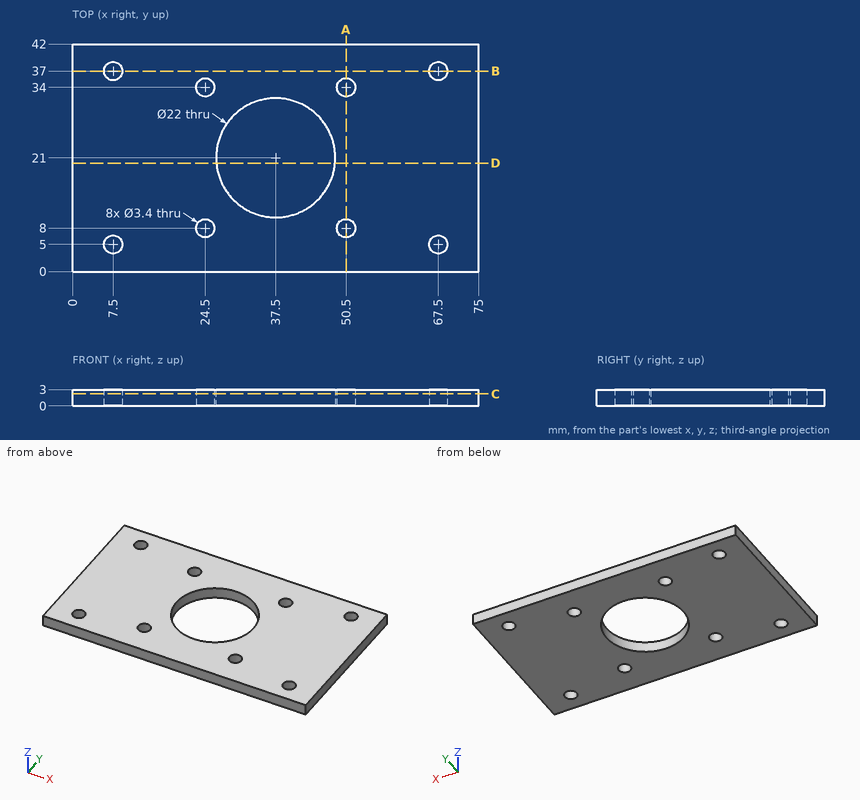
Check sheet for the drawn part. Datum: minimum x, y, z corner. Units: mm. Coordinates: 2 decimals unless noted, no trailing zeros. Loops run counter-clockwise (first coordinate to the right, second up) from the corner with the lowest first, then second, coordinate; pieces in that order, holes last. Notation, with made-up numbers: (40.25, 63.25) -> (51.25, 63.25) arc R27 cw to (51.25, 84.25) -> close; hole circle Ø2 at (4.25, -36). An arc over 180 degrees is marked (long way). Write each question's results on one line, items separated by ' | '.
Item 1: Section check C-C, the plane z = 2.2. Count the separate pieces of the cut face and the enclosed holes in it, plus the area to 3 significant figures.
Found:
separate pieces: 1 | enclosed holes: 9 | area: 2,700 mm2
Item 2: Material ranges on L1, parallel to Y at x = 67.5, z = 1.55; L2, parallel to Y at x = 50.5, z = 0.8; L3, parallel to X at y = 6.5, z = 2.85, recorded low to high.
Found:
L1: y = 0 to 3.3, 6.7 to 35.3, 38.7 to 42 | L2: y = 0 to 6.3, 9.7 to 32.3, 35.7 to 42 | L3: x = 0 to 6.7, 8.3 to 23.7, 25.3 to 49.7, 51.3 to 66.7, 68.3 to 75
Item 3: Section check D-D, the plane y = 20. Enter the section's corners in (x, z), plus the area to 3 significant figures.
Found:
outline: (0, 0) -> (26.55, 0) -> (26.55, 3) -> (0, 3) -> close; (48.45, 0) -> (75, 0) -> (75, 3) -> (48.45, 3) -> close | area: 159 mm2
Item 4: Section check B-B, the plane y = 37. Enter the section's corners in (x, z), plus the area to 3 significant figures.
Found:
outline: (0, 0) -> (5.8, 0) -> (5.8, 3) -> (0, 3) -> close; (9.2, 0) -> (65.8, 0) -> (65.8, 3) -> (9.2, 3) -> close; (69.2, 0) -> (75, 0) -> (75, 3) -> (69.2, 3) -> close | area: 205 mm2
Item 5: Section check A-A, the plane x = 50.5. Enter the section's corners in (y, z).
Found:
outline: (0, 0) -> (6.3, 0) -> (6.3, 3) -> (0, 3) -> close; (9.7, 0) -> (32.3, 0) -> (32.3, 3) -> (9.7, 3) -> close; (35.7, 0) -> (42, 0) -> (42, 3) -> (35.7, 3) -> close
